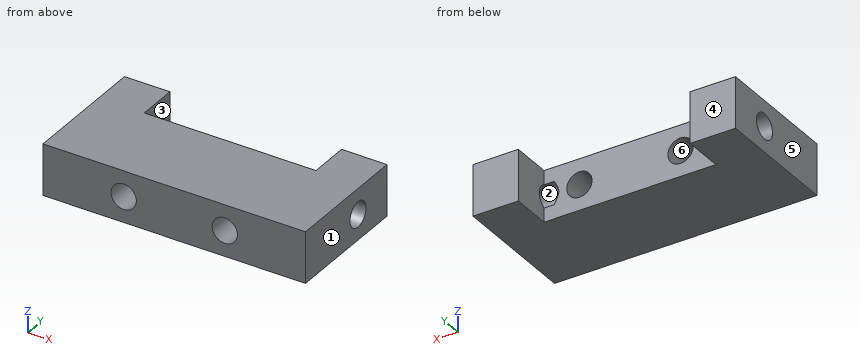
from build123d import *

# Parameters (mm, degrees)
SCHIZZO1_W                   = 25.96
SCHIZZO1_H                   = 12.65
ESTRUSIONE_ESTRUSIONE1_DEPTH = 5.06
SCHIZZO2_W                   = 8.49
SCHIZZO2_H                   = 3.99
TAGLIO_ESTRUSIONE1_DEPTH     = 16.299987745
FORO_FILETTATO_M3X0_5_1_D    = 2.5


with BuildPart() as part:
    # Schizzo1 → Estrusione-Estrusione1 (new body)
    with BuildSketch(Plane.XY):
        Rectangle(SCHIZZO1_W, SCHIZZO1_H)
    extrude(amount=-ESTRUSIONE_ESTRUSIONE1_DEPTH)

    # Schizzo2 → Taglio-Estrusione1 (cut, through all)
    with BuildSketch(Plane.XY):
        with Locations((-4.245, 4.33)):
            Rectangle(SCHIZZO2_W, SCHIZZO2_H)
        with Locations((4.245, 4.33)):
            Rectangle(SCHIZZO2_W, SCHIZZO2_H)
    extrude(amount=-TAGLIO_ESTRUSIONE1_DEPTH, mode=Mode.SUBTRACT)

    # Foro filettato M3x0.5-1 (through all)
    with Locations(Plane(origin=(0, 2.335, 0), x_dir=(1, 0, 0), z_dir=(0, 1, 0))):
        with Locations((-5, 2.53), (5, 2.53)):
            Hole(FORO_FILETTATO_M3X0_5_1_D / 2)

    # Schizzo5 → Foro filettato M3x0.5-2 (revolve, cut)
    with BuildSketch(Plane(origin=(-12.98, 1.825, -2.53), x_dir=(0, 0, 1), z_dir=(0, 1, 0))):
        Polygon((0, 0), (0, 6.251075774), (1.25, 5.5), (1.25, 0), align=None)
    foro_filettato_m3x0_5_2 = revolve(axis=Axis((-19.33, 1.825, -2.53), (1, 0, 0)), mode=Mode.SUBTRACT)

    # Specchia1: Foro filettato M3x0.5-2 across plane
    add(foro_filettato_m3x0_5_2.mirror(Plane(origin=(0, 0, 0), x_dir=(0, 0, 1), z_dir=(1, 0, 0))), mode=Mode.SUBTRACT)


solid = part.part
Geometry check sheet. Reference: the model listing, model coordinates, mm. Face numbers are marked on the shaded views. A direction names the side the tool comes from. Give positions to 0.01 mm unless a question says otherwise; leave off trailing zeros. Write each loop counter-clockwise with the first axis right and the second up, starting at its lowest first coordinate (ties: lowest second). Pieces come first, ordered by that corner, then holes. Notation, with made-up numbers: (-24, 28.5) - (10, 28.5) arc R31 cw to (10, 67.5) - close; hole circle Ø1 at (74, -28.5). An arc over 180 degrees is marked (long way). Put each result on its own line as item: value.
1. Sectioned sample at C-C, the plane y = -3.5. Enter the section's corners in (x, z).
Ans:
outline: (-12.98, -5.06) - (12.98, -5.06) - (12.98, 0) - (-12.98, 0) - close; hole circle Ø2.5 at (-5, -2.53); hole circle Ø2.5 at (5, -2.53)
2. Set-up check for the marked faces 1, 2 and 3: record each of +Z, -Z, +X, -X, +Y, -Y from which the full face is reachable in a straight line by a thin tool's end or side.
Ans:
face 1: +Z, -Z, +X, +Y, -Y
face 2: +X
face 3: +Z, -Z, +Y
3. Draft check along X on the marked faces 4, 5 and 6. Enter one of: +X half, -X half, draft (parallel to the pull), parting line (faces both ways), or undercut.
Ans:
face 4: draft
face 5: -X half
face 6: undercut
4. Sectioned sample at B-B, the plane z = -0.9. Enter the section's corners in (x, y) (3 decimals).
Ans:
outline: (-12.98, -6.325) - (12.98, -6.325) - (12.98, 6.325) - (8.49, 6.325) - (8.49, 2.335) - (-8.49, 2.335) - (-8.49, 6.325) - (-12.98, 6.325) - close
5. Go/stop test with flat-tipped pins: pin 1 (2 mm diameter, centred on y = 1.825, z = -2.53, fed in from +X); pin 2 (1.5 mm diameter, centred on x = -3.5, z = -1, fed in from +Y) (3 decimals). Record where each tip stops, or that it passes through.
Ans:
pin 1: stops at x = 7.33
pin 2: stops at y = 2.335
6. Sectioned sample at A-A, the plane x = 5. Enter the section's corners in (y, z) (3 decimals).
Ans:
outline: (-6.325, -5.06) - (2.335, -5.06) - (2.335, -3.78) - (-6.325, -3.78) - close; (-6.325, -1.28) - (2.335, -1.28) - (2.335, 0) - (-6.325, 0) - close
7. Sectioned sample at D-D, the plane x = -11.5. Enter the section's corners in (y, z) (3 decimals), plus the area to 3 significant figures.
Ans:
outline: (-6.325, -5.06) - (6.325, -5.06) - (6.325, 0) - (-6.325, 0) - close; hole circle Ø2.5 at (1.825, -2.53)
area: 59.1 mm²
8. Thickness scan on line 1 (Z direction, x = -5, y = -3.75); line 2 (X direction, y = 5.5, z = -0.5); line 3 (Y direction, x = 8.8, z = -2.53) (3 decimals). Record the ranges inside material, lowest first.
Ans:
line 1: z = -5.06 to -3.78, -1.28 to 0
line 2: x = -12.98 to -8.49, 8.49 to 12.98
line 3: y = -6.325 to 0.575, 3.075 to 6.325
